The listing builds one solid part. Answer for the finished solid, in the listing's coordinates (mm). A direction names the side the tool comes from. Coordinates: 2 decimals unless noted, no trailing zeros. Order: outer loops, then holes, each group sorted by start corner. A loop starts at its lowest first (then second) coordinate and runs counter-clockwise, first axis right, second up. Notation, with made-up numbers: (84.5, 17) -> (93.5, 17) arc R21 cw to (93.5, 38) -> close; hole circle Ø3 at (60, 84). An arc over 180 degrees is marked (long way). Answer in a Markdown table with one row per item.
```python
from build123d import *

# Parameters (mm, degrees)
F0_R     = 25.4
F1_DEPTH = 101.6
F4_W     = 31.75
F4_H     = 9.525
F6_R     = 5.08
F7_R     = 19.05
F8_DEPTH = 95.25


with BuildPart() as f1:
    # F0 (on Top) → F1 (new body)
    with BuildSketch(Plane.XY):
        Circle(F0_R)
    extrude(amount=F1_DEPTH)

    # F2 (on Front) → F3 (revolve)
    with BuildSketch(Plane.XZ):
        with BuildLine():
            Line((0, -12.8230312839), (0, 0))
            Line((0, 0), (-25.4, 0))
            add(Edge.make_bspline(
                [(-25.4, 0), (-25.4, -7.7090621926), (-11.6054195191, -12.8230312839), (0, -12.8230312839)],
                knots=[0, 0, 0, 0, 28.4532973715, 28.4532973715, 28.4532973715, 28.4532973715], degree=3))
        make_face()
    revolve(axis=Axis((0, 0, -6.411515642), (0, 0, -1)))

    # F4 (on Front) → F5 (revolve)
    with BuildSketch(Plane.XZ):
        with Locations((15.875, 4.7625)):
            Rectangle(F4_W, F4_H)
        with Locations((15.875, 96.8375)):
            Rectangle(F4_W, F4_H)
    revolve(axis=Axis((0, 0, 4.7625), (0, 0, 1)))

    # F6
    f6_edges = [f1.edges().sort_by_distance(p)[0] for p in [
        (-25.4, 0, 92.075),
        (-25.4, 0, 9.525),
    ]]
    fillet(f6_edges, radius=F6_R)

    # F7 (on face) → F8 (cut)
    with BuildSketch(Plane.XY.offset(101.6)):
        Circle(F7_R)
    extrude(amount=-F8_DEPTH, mode=Mode.SUBTRACT)


solid = f1.part
```
(1) Which of the six approach directions +Z, -Z, +X, -X, +Y, -Y give full straight-line access (tool end or side, diameter ignored) to faces 4 (the flat face through (-14, -14, 101.6)), 5 (the cylindrical face through (-5.506, -24.796, 50.293)), 6 (the cylindrical face through (-15.12, -11.59, 54.64)), 7 (the flat face through (14.3, 21.3, 0))?
Check values:
| item | result |
|---|---|
| face 4 | +Z, +X, -X, +Y, -Y |
| face 5 | none |
| face 6 | +Z |
| face 7 | -Z |
(2) Flat-ended cylindrical pins translate along their axes: pin 1 (3 mm diameter, centred on x = 12.5, y = 5.5, fed in from +Z); pin 2 (3 mm diameter, centred on x = 24.5, z = 19, fed in from -Y); pin 3 (1 mm diameter, centred on y = -11, z = 72.5, fed in from +X). Find the tip coordinate at first contact, or state that the pin passes through.
Check values:
| item | result |
|---|---|
| pin 1 | z = 6.35 |
| pin 2 | y = -10.78 |
| pin 3 | x = 23.13 |
(3) Find the intervals of material crossed by line 1 along Z through (x, y) = (-16, -26.5) (3 decimals); line 2 along Y through (x, z) = (0, 64.5); line 3 along Y through (x, z) = (10, 32.5), in increasing order. Write a range as from..to.
Check values:
| item | result |
|---|---|
| line 1 | 0..9.525, 92.075..101.6 |
| line 2 | -25.4..-19.05, 19.05..25.4 |
| line 3 | -23.35..-16.21, 16.21..23.35 |
(4) A cutting plane is placed at A-A, the plane z = 42.5. Determine the outline of the cut face in (x, y).
Check values:
| item | result |
|---|---|
| outline | circle Ø50.8 at (0, 0); hole circle Ø38.1 at (0, 0) |
(5) For a pull along X with two mould halves and no side action, classify faces 1 (the flat face through (11.9, 28.4, 92.075)), 2 (the flat face through (0, 0, 6.35)), 3 (the cylindrical face through (-6.883, -30.995, 4.829)) as released by +X, released by -X, zero draft, split by the parting line, or undercut.
Check values:
| item | result |
|---|---|
| face 1 | zero draft |
| face 2 | undercut |
| face 3 | split by the parting line |
